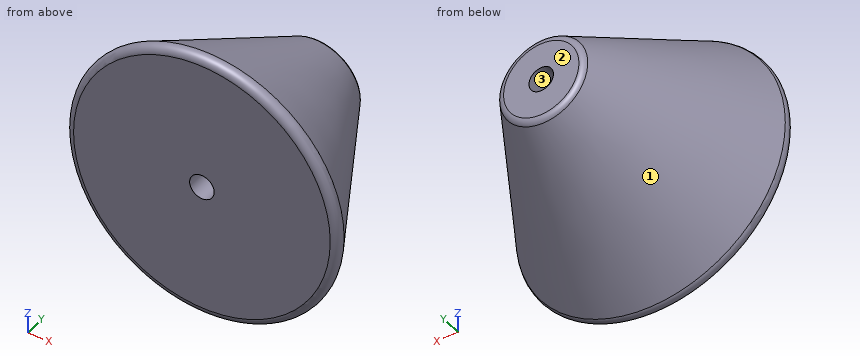
```python
from build123d import *

# Parameters (mm, degrees)
SKETCH1_R           = 57.5
BOSS_EXTRUDE1_DEPTH = 70
BOSS_EXTRUDE1_TAPER = 30
SKETCH3_R           = 5
CUT_EXTRUDE2_DEPTH  = 108.296318842
FILLET1_R           = 3


with BuildPart() as part:
    # Sketch1 → Boss-Extrude1 (new body)
    with BuildSketch(Plane(origin=(0, 0, 0), x_dir=(1, 0, 0), z_dir=(0, 1, 0))):
        Circle(SKETCH1_R)
    extrude(amount=BOSS_EXTRUDE1_DEPTH, taper=BOSS_EXTRUDE1_TAPER)

    # Sketch3 → Cut-Extrude2 (cut, through all)
    with BuildSketch(Plane.XZ):
        with Locations(Location((0, 0, 0), (0, 0, 270))):
            Circle(SKETCH3_R)
    extrude(amount=-CUT_EXTRUDE2_DEPTH, mode=Mode.SUBTRACT)

    # Fillet1
    fillet1_edges = [part.edges().sort_by_distance(p)[0] for p in [
        (-57.5, 0, 0),
        (-17.085481157, 70, 0),
    ]]
    fillet(fillet1_edges, radius=FILLET1_R)


solid = part.part
```
Build history of the part. All positions in model axes, mm. Face numbers are marked on the shaded views. Give positions to 0.01 mm unless a question says otherwise; leave off trailing zeros. Order: outer loops, then holes, each group sorted by start corner. A loop starts at its lowest first (then second) coordinate and runs counter-clockwise, first axis right, second up. Notation, with made-up numbers: M -10,88 L 38,88 A32 ccw 38,124 Z; hole C 55.25,41.5 d10. An arc over 180 degrees is marked long. Write item = value, one per line. Start each with the question number.
(1) Slice it at A-A on x = 0. Write the cut outline in (y, z), plus the area to 3 significant figures.
(2) Two-plate mould, pull along X, no slides. Class the marked faces 1, 2 and 3: released by +X, released by -X, zero draft, split by the parting line, or undercut.
(3) Probe L1, parallel to X at y = 52, z = -0.5; L2, parallel to X at y = 12, z = 34.5; L3, parallel to X at y = 4.5, z = 17. List the from-to ranges inside material, lowest first. Write a range as [from, to].
(4) Pin check, flat tips, straight feed: pin 1 Ø2 at (x, z) = (39, -11.5) entering from +Y; pin 2 Ø1.5 at (x, y) = (-30.5, 40.5) entering from +Z; pin 3 Ø8 at (x, z) = (29.5, 37) entering from -Y; pin 4 Ø3 at (x, y) = (4.5, 48) entering from -Z. Stop position of each tip, or through.
(5) Slice it at B-B on y = 9. Write the cut outline in (x, z), plus the area to 3 significant figures.
(6) Slice it at C-C on y = 27.5. Write the cut outline in (x, z), plus the area to 3 significant figures.
Responses:
q1.outline = M 0,-52.3 A3 ccw 4.5,-54.9 L 68.5,-17.95 A3 ccw 70,-15.35 L 70,-5 L 0,-5 Z; M 0,5 L 70,5 L 70,15.35 A3 ccw 68.5,17.95 L 4.5,54.9 A3 ccw 0,52.3 Z
q1.area = 4,510 mm2
q2.face_1 = split by the parting line
q2.face_2 = zero draft
q2.face_3 = undercut
q3.L1 = [-27.47, -4.97], [4.97, 27.47]
q3.L2 = [-36.98, 36.98]
q3.L3 = [-52.2, 52.2]
q4.pin_1 = 30.9
q4.pin_2 = 16.97
q4.pin_3 = 0
q4.pin_4 = -30.35
q5.outline = C 0,0 d104.61; hole C 0,0 d10
q5.area = 8,520 mm2
q6.outline = C 0,0 d83.25; hole C 0,0 d10
q6.area = 5,360 mm2
